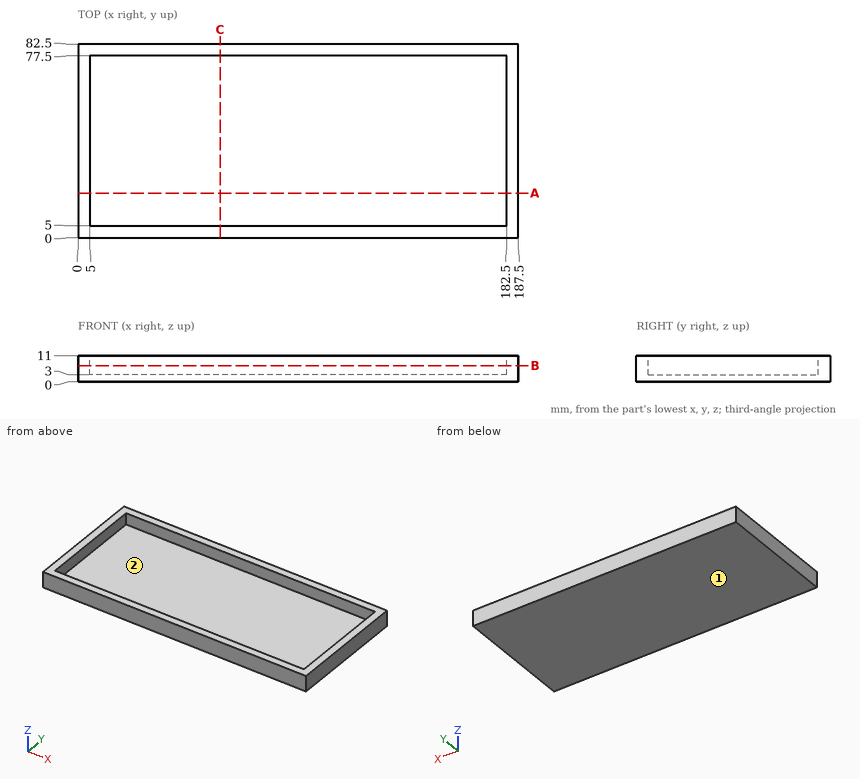
Could you check a few things on this drawing? It's one solid part, dimensions in mm from its lowest x, y, z. Round coordinates to 2 decimals unless told otherwise and drop trailing zeros. Order: outer loops, then holes, each group sorted by start corner. A loop starts at its lowest first (then second) coordinate and runs counter-clockwise, first axis right, second up.
(1) Imagine slicing it at B-B (z = 6.75). Write out the boundary of the cut face in (x, y), plus the area to 3 significant figures.
Response values:
outline: (0, 0) - (187.5, 0) - (187.5, 82.5) - (0, 82.5) - close; hole (5, 5) - (182.5, 5) - (182.5, 77.5) - (5, 77.5) - close
area: 2,600 mm2
(2) I'm going to push flat-ended pins straight in: pin 1 (2.5 mm diameter, centred on x = 55, z = 8, fed in from -Y); pin 2 (2 mm diameter, centred on x = 116.5, y = 12.5, fed in from +Z). Where does each tip first touch, or does it pass through?
Response values:
pin 1: stops at y = 0
pin 2: stops at z = 3
(3) Please list where these lines run through material, in increasing order: line 1 along X through (y, z) = (36, 5.5); line 2 along Y through (x, z) = (106, 3.75); line 3 along Z through (x, y) = (62.5, 51.5).
Response values:
line 1: x = 0 to 5, 182.5 to 187.5
line 2: y = 0 to 5, 77.5 to 82.5
line 3: z = 0 to 3
(4) Imagine slicing it at C-C (x = 60.5). Write out the boundary of the cut face in (y, z), plus the area to 4 significant figures.
Response values:
outline: (0, 0) - (82.5, 0) - (82.5, 11) - (77.5, 11) - (77.5, 3) - (5, 3) - (5, 11) - (0, 11) - close
area: 327.5 mm2
(5) Imagine slicing it at A-A (y = 19). Write out the boundary of the cut face in (x, z), plus the area to 4 significant figures.
Response values:
outline: (0, 0) - (187.5, 0) - (187.5, 11) - (182.5, 11) - (182.5, 3) - (5, 3) - (5, 11) - (0, 11) - close
area: 642.5 mm2
(6) If we mould it in two halves opening along Y, with no side actions, what happens to the marked faces 1 and 2? For each: released by +Y, released by -Y, zero draft, split by the parting line, or undercut.
Response values:
face 1: zero draft
face 2: undercut
